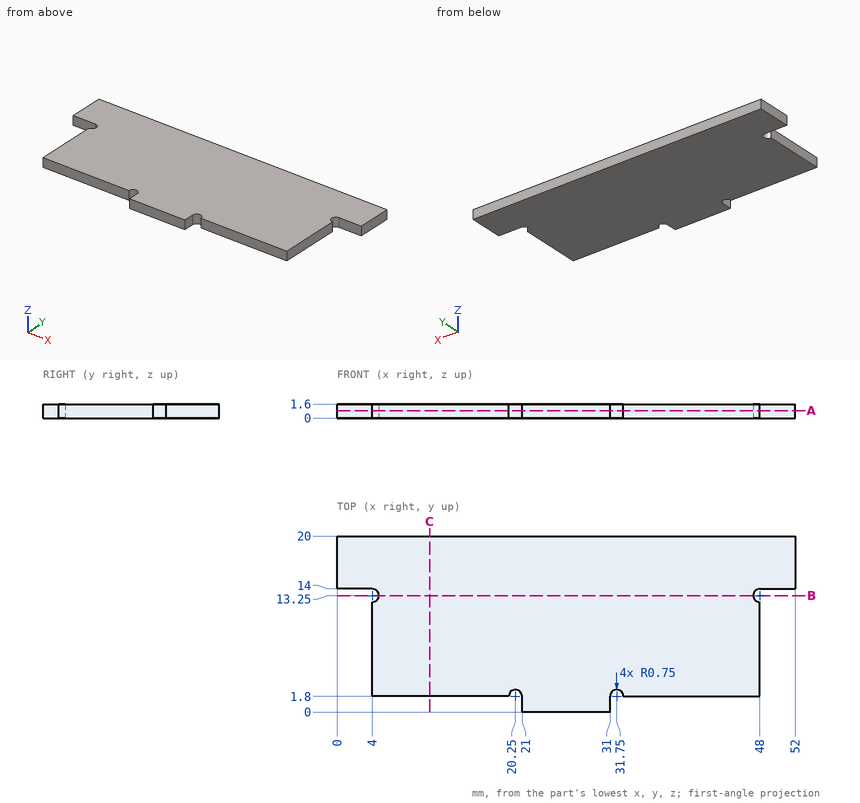
Answer from the drawing. Dimensions are ordinates in mm from the lowest x, y and z of the part. Coordinates: 2 decimals unless noted, no trailing zeros. Loops run counter-clockwise (first coordinate to the right, second up) from the corner with the lowest first, then second, coordinate; pieces in that order, holes last.
Q1. The part is cut by section B-B on y = 13.25. Write down the section's boundary in (x, z).
Q2. Each of these flat-tipped pins is pushed along its axis until it touches: pin 1 Ø3 at (x, y) = (19, 11.5) entering from -Z; pin 2 Ø0.8 at (x, z) = (49.5, 0.5) entering from -Y; pin 3 Ø0.8 at (y, z) = (8.5, 1) entering from +X. Where does it stop, or does it pass through?
Q3. The part is cut by section C-C on x = 10.5. Write down the section's boundary in (y, z).
Q4. The part is cut by section A-A on z = 0.85. Write down the section's boundary in (x, y).
Q5. Consider probe 1 along X at (y, z) = (2, 0.3); probe 2 along X at (y, z) = (9.5, 1.4); probe 3 along Y at (x, z) = (11.5, 0.7). Determine where each line is inside the solid, lowest interval first.
Results below:
1. outline: (4.75, 0) - (47.25, 0) - (47.25, 1.6) - (4.75, 1.6) - close
2. pin 1: stops at z = 0
2. pin 2: stops at y = 14
2. pin 3: stops at x = 48
3. outline: (1.8, 0) - (20, 0) - (20, 1.6) - (1.8, 1.6) - close
4. outline: (0, 14) - (4, 14) arc R0.75 cw to (4, 12.5) - (4, 1.8) - (19.5, 1.8) arc R0.75 cw to (21, 1.8) - (21, 0) - (31, 0) - (31, 1.8) arc R0.75 cw to (32.5, 1.8) - (48, 1.8) - (48, 12.5) arc R0.75 cw to (48, 14) - (52, 14) - (52, 20) - (0, 20) - close
5. probe 1: x = 4 to 19.53, 20.97 to 31.03, 32.47 to 48
5. probe 2: x = 4 to 48
5. probe 3: y = 1.8 to 20
